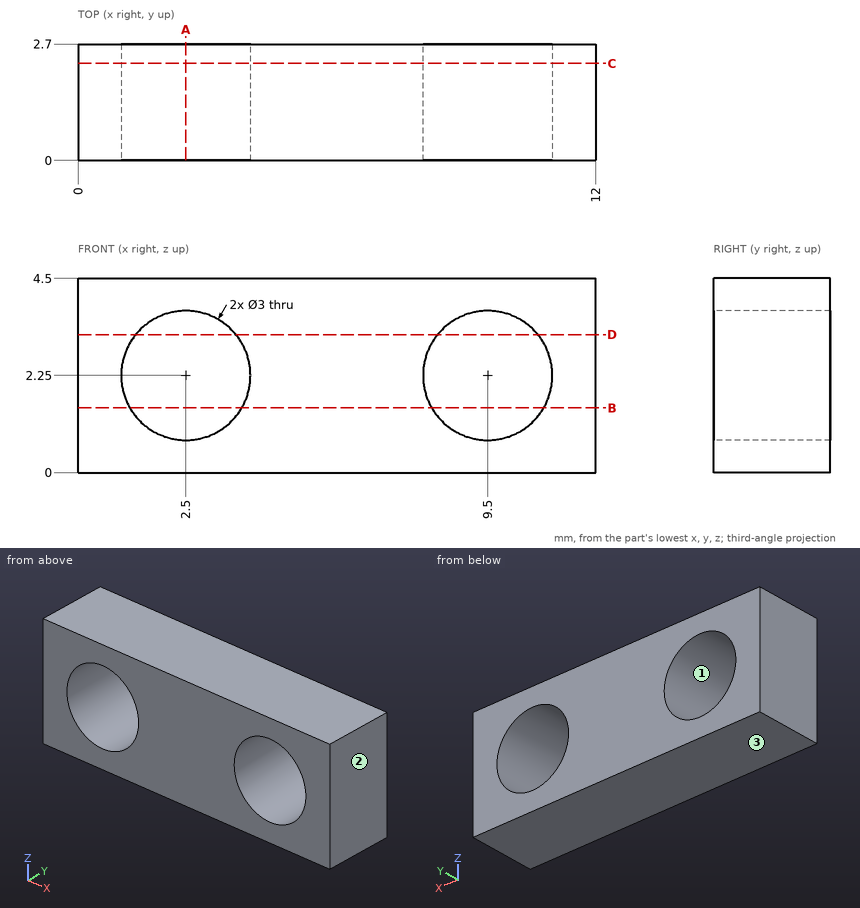
Design review of the part shown in the three views and the two pictorial views. Dimensions are in mm from the part's minimum x, y and z. Round coordinates to 2 decimals unless told otherwise and drop trailing zeros. Loops run counter-clockwise (first coordinate to the right, second up) from the corner with the lowest first, then second, coordinate; pieces in that order, holes last. Notation, with made-up numbers: M 1.5,28.25 L 38.5,28.25 A9 ccw 38.5,45.25 Z; hole C 66.5,20.25 d3. An arc over 180 degrees is marked long. Write item = value, one per line.
Item 1: Take a section at B-B on z = 1.5. Write out the cut boundary in (x, y).
Return value:
outline = M 0,0 L 1.2,0 L 1.2,2.7 L 0,2.7 Z; M 3.8,0 L 8.2,0 L 8.2,2.7 L 3.8,2.7 Z; M 10.8,0 L 12,0 L 12,2.7 L 10.8,2.7 Z
Item 2: For line 1 (Z direction, x = 2.5, y = 1.7); line 2 (X direction, y = 0.45, z = 3); line 3 (X direction, y = 2.55, z = 2.6), list the stretches that pass through material, from the lowest coordinate up. Write a range as [from, to].
Return value:
line_1 = [0, 0.75], [3.75, 4.5]
line_2 = [0, 1.2], [3.8, 8.2], [10.8, 12]
line_3 = [0, 1.04], [3.96, 8.04], [10.96, 12]
Item 3: The part is to be moulded in two halves that separate along Z. For the marked faces 1, 2 and 3, say which applies: released by +Z, released by -Z, zero draft, split by the parting line, or undercut.
Return value:
face_1 = undercut
face_2 = zero draft
face_3 = released by -Z
Item 4: Take a section at D-D on z = 3.2. Write out the cut boundary in (x, y).
Return value:
outline = M 0,0 L 1.34,0 L 1.34,2.7 L 0,2.7 Z; M 3.66,0 L 8.34,0 L 8.34,2.7 L 3.66,2.7 Z; M 10.66,0 L 12,0 L 12,2.7 L 10.66,2.7 Z
Item 5: Take a section at A-A on x = 2.5. Write out the cut boundary in (y, z), then the cut area to 3 significant figures.
Return value:
outline = M 0,0 L 2.7,0 L 2.7,0.75 L 0,0.75 Z; M 0,3.75 L 2.7,3.75 L 2.7,4.5 L 0,4.5 Z
area = 4.05 mm2
Item 6: Take a section at C-C on y = 2.25. Write out the cut boundary in (x, z), then the cut area to 3 significant figures.
Return value:
outline = M 0,0 L 12,0 L 12,4.5 L 0,4.5 Z; hole C 2.5,2.25 d3; hole C 9.5,2.25 d3
area = 39.9 mm2
